Work out the finished part from the listing and answer in its coordinate system (mm). Face numbers are marked on the shaded views. A direction names the side the tool comes from. Round coordinates to 2 decimals unless told otherwise and drop trailing zeros. Loops run counter-clockwise (first coordinate to the right, second up) from the corner with the lowest first, then second, coordinate; pieces in that order, holes last. Notation, with made-up numbers: (11.25, 37) -> (51.25, 37) arc R16 cw to (51.25, 44) -> close; hole circle Ø1 at (13, -4). An arc over 180 degrees is marked (long way). Use one line per item in the form item = value.
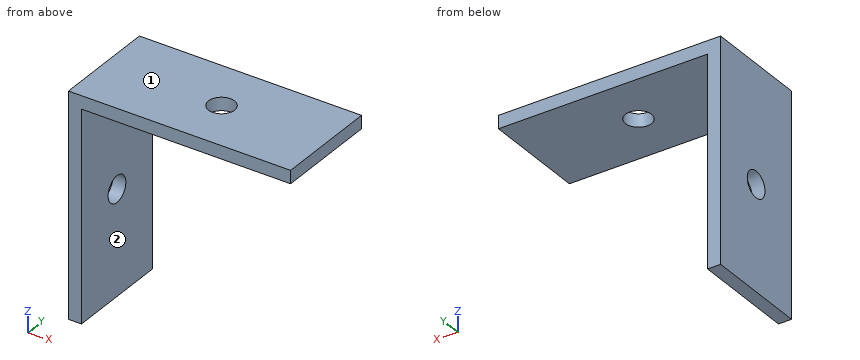
Autodesk Inventor part; units mm, degrees
ref_plane "YZ Plane" through (0, 0, 0) normal (1, 0, 0) x (0, 1, 0)
ref_plane "XZ Plane" through (0, 0, 0) normal (0, 1, 0) x (-1, 0, 0)
ref_plane "XY Plane" through (0, 0, 0) normal (0, 0, 1) x (1, 0, 0)
sketch "Sketch1" plane through (0, 0, 0) normal (1, 0, 0) x (0, 1, 0)
  line L0 (0, 0) -> (12.7, 0)
  line L1 (12.7, 0) -> (12.7, 25.4)
  line L2 (12.7, 25.4) -> (0, 25.4)
  line L3 (0, 25.4) -> (0, 0)
  dimension "d0" = 25.4
  dimension "d1" = 12.7
extrude "Extrusion1" add sketch "Sketch1" along normal blind 1.5875
sketch "Sketch2" plane through (1.5875, 0, 0) normal (1, 0, 0) x (0, 0, -1)
  line L0 (0, 0) -> (0, 12.7)
  line L1 (0, 12.7) -> (-25.4, 12.7)
  line L2 (-25.4, 12.7) -> (-25.4, 0)
  line L3 (-25.4, 0) -> (0, 0)
sketch "Sketch3" plane through (0, 0, 0) normal (-1, 0, 0) x (0, 0, 1)
  line L0 (25.4, 12.7) -> (26.9875, 12.7)
  line L1 (26.9875, 12.7) -> (26.9875, 0)
  line L2 (26.9875, 0) -> (25.4, 0)
  line L3 (25.4, 0) -> (25.4, 12.7)
  dimension "d4" = 1.5875
extrude "Extrusion2" add sketch "Sketch3" against normal blind 26.9875
sketch "Sketch4" plane through (1.5875, 0, 0) normal (1, 0, 0) x (0, 0, -1)
  line L0 (0, 0) -> (0, 12.7)
  line L1 (-25.4, 0) -> (0, 0)
  point P0 (-12.7, 6.35)
  dimension "d8" = 6.35
  dimension "d9" = 12.7
sketch "Sketch5" plane through (26.9875, 12.7, 25.4) normal (0, 0, -1) x (-1, 0, 0)
  line L0 (0, -12.7) -> (0, 0)
  line L1 (25.4, -12.7) -> (0, -12.7)
  point P0 (26.9875, -12.7)
  point P1 (12.7, -6.35)
  dimension "d10" = 6.35
  dimension "d11" = 12.7
hole "Hole1" at (14.2875, 6.35, 25.4) direction (0, 0, 1) diameter 3.175 depth 25.4 tip angle 118
hole "Hole2" at (1.5875, 6.35, 12.7) direction (-1, 0, 0) diameter 3.175 depth 25.4 tip angle 118
properties part number "SideSupport" material "Aluminum 6061"
(1) Find section C-C, the plane x = 15.25. Write down the section's boundary in (y, z), then the cut area to 3 significant figures.
Completed:
outline = (0, 25.4) -> (5.09, 25.4) -> (5.09, 26.99) -> (0, 26.99) -> close; (7.61, 25.4) -> (12.7, 25.4) -> (12.7, 26.99) -> (7.61, 26.99) -> close
area = 16.2 mm2
(2) Find section D-D, the plane y = 9.5. Write down the section's boundary in (x, z), then the cut area to 3 significant figures.
Completed:
outline = (0, 0) -> (1.59, 0) -> (1.59, 25.4) -> (26.99, 25.4) -> (26.99, 26.99) -> (0, 26.99) -> close
area = 83.2 mm2
(3) For the marked faces 1 and 2, determine the directions among +Z, -Z, +X, -X, +Y, -Y from which every point of the face is accessible in a straight line to the end or side of a thin tool.
Completed:
face_1 = +Z, +X, -X, +Y, -Y
face_2 = -Z, +X, +Y, -Y
(4) Given P1, Ø6.5, axis at y = 9, z = 16.5, coming from the +X side, flat-ended and moving along its own axis, determine where the tip first touches the part or whether it passes through.
Completed:
P1 = 1.59
(5) Find section B-B, the plane y = 6.35. Write down the section's boundary in (x, z) (1 decimal).
Completed:
outline = (0, 0) -> (1.6, 0) -> (1.6, 11.1) -> (0, 11.1) -> close; (0, 14.3) -> (1.6, 14.3) -> (1.6, 25.4) -> (12.7, 25.4) -> (12.7, 27) -> (0, 27) -> close; (15.9, 25.4) -> (27, 25.4) -> (27, 27) -> (15.9, 27) -> close
(6) Find section A-A, the plane z = 12.7. Write down the section's boundary in (x, y), then the cut area to 3 significant figures.
Completed:
outline = (0, 0) -> (1.59, 0) -> (1.59, 4.76) -> (0, 4.76) -> close; (0, 7.94) -> (1.59, 7.94) -> (1.59, 12.7) -> (0, 12.7) -> close
area = 15.1 mm2
(7) Consider L1, parallel to Y at x = 0.85, z = 12.7; L2, parallel to X at y = 6.35, z = 26.35 (1 decimal); L3, parallel to Z at x = 1.35, y = 6.35. Determine where each line is inside the solid, lowest interval first.
Completed:
L1 = 0 to 4.76, 7.94 to 12.7
L2 = 0 to 12.7, 15.9 to 27
L3 = 0 to 11.11, 14.29 to 26.99
